```python
from build123d import *

# Parameters (mm, degrees)
SKETCH1_W           = 286.300000032
SKETCH1_H           = 263.675
BOSS_EXTRUDE1_DEPTH = 1.5875
SKETCH4_W           = 3.175
SKETCH4_H           = 38.1
SKETCH4_W_2         = 38.1
SKETCH4_H_2         = 6.35
BOSS_EXTRUDE2_DEPTH = 3.175
SKETCH3_W           = 50.8
SKETCH3_H           = 31.75
CUT_EXTRUDE2_DEPTH  = 3.175


with BuildPart() as part:
    # Sketch1 → Boss-Extrude1 (new body, symmetric)
    with BuildSketch(Plane.XY):
        with Locations((-144.737500016, 135.0125)):
            Rectangle(SKETCH1_W, SKETCH1_H)
    extrude(amount=BOSS_EXTRUDE1_DEPTH, both=True)

    # Sketch4 → Boss-Extrude2 (add)
    with BuildSketch(Plane.XY.offset(1.5875)):
        with Locations((-289.475000032, 200.93125)):
            Rectangle(SKETCH4_W, SKETCH4_H)
        with Locations((-289.475000032, 135.0125)):
            Rectangle(SKETCH4_W, SKETCH4_H)
        with Locations((-289.475000032, 69.09375)):
            Rectangle(SKETCH4_W, SKETCH4_H)
        with Locations((0, 200.93125)):
            Rectangle(SKETCH4_W, SKETCH4_H)
        with Locations((0, 135.0125)):
            Rectangle(SKETCH4_W, SKETCH4_H)
        with Locations((0, 69.09375)):
            Rectangle(SKETCH4_W, SKETCH4_H)
        with Locations((-217.106250024, 0)):
            Rectangle(SKETCH4_W_2, SKETCH4_H_2)
        with Locations((-144.737500016, 0)):
            Rectangle(SKETCH4_W_2, SKETCH4_H_2)
        with Locations((-72.368750008, 0)):
            Rectangle(SKETCH4_W_2, SKETCH4_H_2)
    extrude(amount=-BOSS_EXTRUDE2_DEPTH)

    # Sketch3 → Cut-Extrude2 (cut)
    with BuildSketch(Plane.XY.offset(1.5875)):
        with Locations((-26.9875, 250.975)):
            Rectangle(SKETCH3_W, SKETCH3_H)
    extrude(amount=-CUT_EXTRUDE2_DEPTH, mode=Mode.SUBTRACT)


solid = part.part
```
Geometry: final body of the model. Coordinates: model frame, mm. Give positions to 0.01 mm unless a question says otherwise; leave off trailing zeros. Loops run counter-clockwise (first coordinate to the right, second up) from the corner with the lowest first, then second, coordinate; pieces in that order, holes last. Notation, with made-up numbers: (-11, 47) - (31, 47) arc R12 ccw to (31, 52) - close; hole circle Ø7 at (-12.5, -11). An arc over 180 degrees is marked (long way). Answer as CSV lines item,"result". Start each with the question number.
(1) Ray query, line 1 along X through (y, z) = (171.5, -1.2); line 2 along Y through (x, z) = (-21, -0.6) (3 decimals); line 3 along Y through (x, z) = (-166.5, 1) (3 decimals). Return the intervals inside material, ascending. Write a range as [from, to].
(2) Pin query (flat end, axial travel): P1, Ø1, axis at x = -164.5, z = 0.5, coming from the -Y side (3 decimals); P2, Ø1, axis at x = -290, z = 0.5, coming from the +Y side; P3, Ø1, axis at y = 99, z = 0, coming from the -X side. Return the tip coordinate at first contact, or that it passes through.
(3) Section query B-B (y = 173.5). Output: boundary loops of the cut face in (x, z), and give its area (3 significant figures).
(4) Section query A-A (x = -24.5). Output: boundary loops of the cut face in (y, z) (1 decimal).
Worked answers:
1,line 1,"x = [-287.89, -1.59]"
1,line 2,"y = [3.175, 235.1]"
1,line 3,"y = [3.175, 266.85]"
2,P1,"stops at y = 3.175"
2,P2,"stops at y = 219.98"
2,P3,"stops at x = -287.89"
3,outline,"(-287.89, -1.59) - (-1.59, -1.59) - (-1.59, 1.59) - (-287.89, 1.59) - close"
3,area,"909 mm^2"
4,outline,"(3.2, -1.6) - (235.1, -1.6) - (235.1, 1.6) - (3.2, 1.6) - close"
